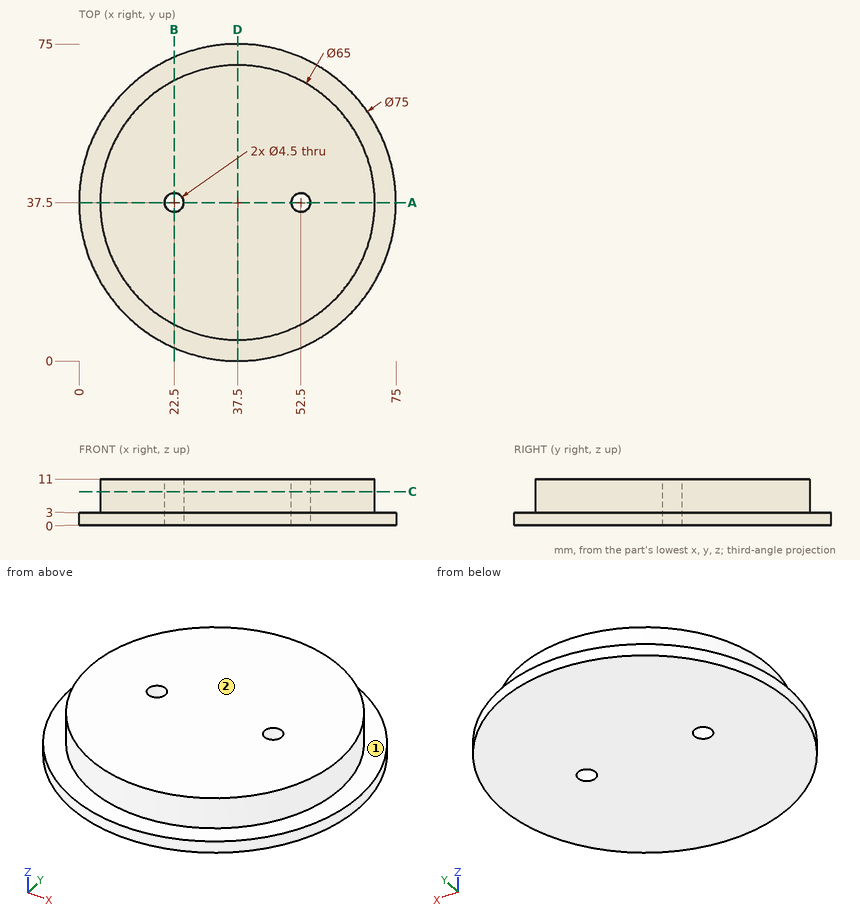
Print and shaded views of the part. All mm, measured from the part's lowest x, y and z. A direction names the side the tool comes from. Coordinates: 2 decimals unless noted, no trailing zeros. Loops run counter-clockwise (first coordinate to the right, second up) from the corner with the lowest first, then second, coordinate; pieces in that order, holes last. Notation, with made-up numbers: M 82,67.25 L 92,67.25 A31 ccw 92,93.25 Z; hole C -21.5,84 d11. An arc over 180 degrees is marked long. Use a Markdown table: item, result. Add a question column.
Q1. Cut at D-D (x = 37.5). Write the cut outline in (y, z).
Q2. Cut at B-B (x = 22.5). Write the cut outline in (y, z), and give its area (3 significant figures).
Q3. Pin check, flat tips, straight feed: P1, Ø5, axis at y = 45.5, z = 6.5, coming from the -X side; P2, Ø2, axis at y = 18, z = 6.5, coming from the -X side; P3, Ø6, axis at x = 52.5, y = 37.5, coming from the -Z side; P4, Ø2.5, axis at x = 22.5, y = 37.5, coming from the +Z side. Stop position of each tip, or through.
Q4. Which spindle directions (+Z, -Z, +X, -X, +Y, -Y) get a long thin tool onto all of the face, cutting with end or side? Do the marked faces 1 and 2. Say none if no direction does.
Q5. Probe L1, parallel to Z at x = 66, y = 20; L2, parallel to Y at x = 52.5, z = 8; L3, parallel to Y at x = 41, z = 9.5. List the from-to ranges inside material, lowest first.
Q6. Cut at C-C (z = 8). Write the cut outline in (x, y), and give its area (3 significant figures).
Q7. Cut at A-A (y = 37.5). Write the cut outline in (x, z).
Worked out:
| question | item | result |
|---|---|---|
| 1 | outline | M 0,0 L 75,0 L 75,3 L 70,3 L 70,11 L 5,11 L 5,3 L 0,3 Z |
| 2 | outline | M 3.13,0 L 35.25,0 L 35.25,11 L 8.67,11 L 8.67,3 L 3.13,3 Z; M 39.75,0 L 71.87,0 L 71.87,3 L 66.33,3 L 66.33,11 L 39.75,11 Z |
| 2 | area | 618 mm2 |
| 3 | P1 | stops at x = 5.47 |
| 3 | P2 | stops at x = 10.78 |
| 3 | P3 | stops at z = 0 |
| 3 | P4 | passes through |
| 4 | face 1 | +Z |
| 4 | face 2 | +Z, +X, -X, +Y, -Y |
| 5 | L1 | z = 0 to 3 |
| 5 | L2 | y = 8.67 to 35.25, 39.75 to 66.33 |
| 5 | L3 | y = 5.19 to 69.81 |
| 6 | outline | C 37.5,37.5 d65; hole C 22.5,37.5 d4.5; hole C 52.5,37.5 d4.5 |
| 6 | area | 3,290 mm2 |
| 7 | outline | M 0,0 L 20.25,0 L 20.25,11 L 5,11 L 5,3 L 0,3 Z; M 24.75,0 L 50.25,0 L 50.25,11 L 24.75,11 Z; M 54.75,0 L 75,0 L 75,3 L 70,3 L 70,11 L 54.75,11 Z |
